```python
from build123d import *

# Parameters (mm, degrees)
SKETCH1_W               = 700
SKETCH1_H               = 450
BOSS_EXTRUDE1_DEPTH     = 1000
SKETCH2_W               = 650
SKETCH2_H               = 600
CUT_EXTRUDE1_DEPTH      = 250
CUT_EXTRUDE1_DEPTH_BACK = 250
SKETCH3_W               = 650
SKETCH3_H               = 350
CUT_EXTRUDE2_DEPTH      = 250
CUT_EXTRUDE2_DEPTH_BACK = 250
SKETCH4_W               = 400
SKETCH4_H               = 600
CUT_EXTRUDE3_DEPTH      = 400
CUT_EXTRUDE3_DEPTH_BACK = 400
SKETCH5_W               = 400
SKETCH5_H               = 350
CUT_EXTRUDE4_DEPTH      = 400
CUT_EXTRUDE4_DEPTH_BACK = 400
ESBO_O1_R               = 8
ESBO_O1_W               = 150
ESBO_O1_H               = 110
CORTE_EXTRUS_O1_DEPTH   = 50
ESBO_O2_W               = 250
ESBO_O2_H               = 70
CORTE_EXTRUS_O2_DEPTH   = 26
ESBO_O3_R               = 6.25
CORTE_EXTRUS_O3_DEPTH   = 10
ESBO_O5_R               = 3
CORTE_EXTRUS_O4_DEPTH   = 26
ESBO_O7_R               = 6
CORTE_EXTRUS_O5_DEPTH   = 5


with BuildPart() as part:
    # Sketch1 → Boss-Extrude1 (new body)
    with BuildSketch(Plane(origin=(0, 0, 0), x_dir=(1, 0, 0), z_dir=(0, 1, 0))):
        Rectangle(SKETCH1_W, SKETCH1_H)
    extrude(amount=BOSS_EXTRUDE1_DEPTH)

    # Sketch2 → Cut-Extrude1 (cut, two sides)
    with BuildSketch(Plane.XY) as cut_extrude1_sk:
        with Locations((0, 675)):
            Rectangle(SKETCH2_W, SKETCH2_H)
    extrude(amount=CUT_EXTRUDE1_DEPTH, mode=Mode.SUBTRACT)
    extrude(cut_extrude1_sk.sketch, amount=-CUT_EXTRUDE1_DEPTH_BACK, mode=Mode.SUBTRACT)

    # Sketch3 → Cut-Extrude2 (cut, two sides)
    with BuildSketch(Plane.XY) as cut_extrude2_sk:
        with Locations((0, 175)):
            Rectangle(SKETCH3_W, SKETCH3_H)
    extrude(amount=CUT_EXTRUDE2_DEPTH, mode=Mode.SUBTRACT)
    extrude(cut_extrude2_sk.sketch, amount=-CUT_EXTRUDE2_DEPTH_BACK, mode=Mode.SUBTRACT)

    # Sketch4 → Cut-Extrude3 (cut, two sides)
    with BuildSketch(Plane(origin=(0, 0, 0), x_dir=(0, 0, -1), z_dir=(1, 0, 0))) as cut_extrude3_sk:
        with Locations((0, 675)):
            Rectangle(SKETCH4_W, SKETCH4_H)
    extrude(amount=CUT_EXTRUDE3_DEPTH, mode=Mode.SUBTRACT)
    extrude(cut_extrude3_sk.sketch, amount=-CUT_EXTRUDE3_DEPTH_BACK, mode=Mode.SUBTRACT)

    # Sketch5 → Cut-Extrude4 (cut, two sides)
    with BuildSketch(Plane(origin=(0, 0, 0), x_dir=(0, 0, -1), z_dir=(1, 0, 0))) as cut_extrude4_sk:
        with Locations((0, 175)):
            Rectangle(SKETCH5_W, SKETCH5_H)
    extrude(amount=CUT_EXTRUDE4_DEPTH, mode=Mode.SUBTRACT)
    extrude(cut_extrude4_sk.sketch, amount=-CUT_EXTRUDE4_DEPTH_BACK, mode=Mode.SUBTRACT)

    # Esboço1 → Corte-extrusão1 (cut)
    with BuildSketch(Plane(origin=(0, 1000, 0), x_dir=(1, 0, 0), z_dir=(0, 1, 0))):
        with Locations((-100.84, 100)):
            Circle(ESBO_O1_R)
        with Locations((-230, 100)):
            Circle(ESBO_O1_R)
        with Locations((-230, -74.37)):
            Circle(ESBO_O1_R)
        with Locations((0, -74.37)):
            Circle(ESBO_O1_R)
        with Locations((230, -74.37)):
            Circle(ESBO_O1_R)
        with Locations((-165.42, 10.42)):
            Rectangle(ESBO_O1_W, ESBO_O1_H)
    extrude(amount=-CORTE_EXTRUS_O1_DEPTH, mode=Mode.SUBTRACT)

    # Esboço2 → Corte-extrusão2 (cut, through all)
    with BuildSketch(Plane(origin=(0, 975, 0), x_dir=(-1, 0, 0), z_dir=(0, -1, 0))):
        with Locations((-170, -105)):
            Rectangle(ESBO_O2_W, ESBO_O2_H)
    extrude(amount=-CORTE_EXTRUS_O2_DEPTH, mode=Mode.SUBTRACT)

    # Esboço3 → Corte-extrusão3 (cut)
    with BuildSketch(Plane(origin=(0, 1000, 0), x_dir=(1, 0, 0), z_dir=(0, 1, 0))):
        with Locations((270, -13.671274916)):
            Circle(ESBO_O3_R)
        with Locations((270, 96.328725084)):
            Circle(ESBO_O3_R)
        with Locations((125, 96.328725084)):
            Circle(ESBO_O3_R)
        with Locations((125, -13.671274916)):
            Circle(ESBO_O3_R)
    extrude(amount=-CORTE_EXTRUS_O3_DEPTH, mode=Mode.SUBTRACT)

    # Esboço5 → Corte-extrusão4 (cut, through all)
    with BuildSketch(Plane.XZ.offset(-975)):
        with Locations((93, -180)):
            Circle(ESBO_O5_R)
        with Locations((93, -113.3)):
            Circle(ESBO_O5_R)
        with Locations((230, -113.3)):
            Circle(ESBO_O5_R)
        with Locations((230, -180)):
            Circle(ESBO_O5_R)
    extrude(amount=-CORTE_EXTRUS_O4_DEPTH, mode=Mode.SUBTRACT)

    # Esboço7 → Corte-extrusão5 (cut)
    with BuildSketch(Plane(origin=(0, 1000, 0), x_dir=(1, 0, 0), z_dir=(0, 1, 0))):
        with Locations((315, 75)):
            Circle(ESBO_O7_R)
    extrude(amount=-CORTE_EXTRUS_O5_DEPTH, mode=Mode.SUBTRACT)


solid = part.part
```
Design review of the part built by this model. Coordinates are the model's own, in mm. A direction names the side the tool comes from. Coordinates: 2 decimals unless noted, no trailing zeros. Write each loop counter-clockwise with the first axis right and the second up, starting at its lowest first coordinate (ties: lowest second). Pieces come first, ordered by that corner, then holes.
1) To check wall thickness, follow L1, parallel to Z at x = 230, y = 987.25; L2, parallel to Z at x = 315, y = 998; L3, parallel to X at y = 991.25, z = 74.37. State the ranges of each line that lie inside material, in increasing order.
2) Add section A-A (x = -169.5). Write out the cut boundary in (y, z).
3) Insertion check: pin 1 (21 mm diameter, centred on x = -100.84, z = -100, fed in from -Y); pin 2 (4 mm diameter, centred on x = 267.5, z = 15.5, fed in from +Y). Each pin has a flat end and moves straight along its axis. Give the tip position at first contact, or say it passes through.
4) Add section D-D (y = 730). Write out the cut boundary in (x, z), plus the area to 3 significant figures.
5) Machinability: for faces 1 (the flat face through (-337, 173, -200)), 2 (the flat face through (337, 671, -200)), 3 (the flat face through (325, 671, 212)), which of the approach directions +Z, -Z, +X, -X, +Y, -Y give a long, thin tool a straight path to every point of the face, cutting with its end or side? Answer none if there is none.
6) Add section B-B (x = -74.5). Write out the cut boundary in (y, z), plus the area to 3 significant figures.
7) Add section C-C (z = 102.5). Write out the cut boundary in (x, y).
8) Mouldability with a two-part tool opening along Y and no side actions: class faces 4 (the flat face through (-337, 671, -200)), 5 (the flat face through (-338, 0, 212)), 6 (the flat face through (337, 173, -200)) as +Y half, -Y half, draft (parallel to the pull), parting line (faces both ways), or undercut.
Check result:
1. L1: z = -225 to -183, -177 to -116.3, -110.3 to 66.37, 140 to 225
1. L2: z = -225 to -81, -69 to 225
1. L3: x = -350 to -238, -222 to -8, 8 to 45, 295 to 350
2. outline: (350, -225) - (375, -225) - (375, 225) - (350, 225) - close; (975, -225) - (1000, -225) - (1000, -65.42) - (975, -65.42) - close; (975, 44.58) - (1000, 44.58) - (1000, 225) - (975, 225) - close
3. pin 1: stops at y = 350
3. pin 2: stops at y = 990
4. outline: (-350, -225) - (-325, -225) - (-325, -200) - (-350, -200) - close; (-350, 200) - (-325, 200) - (-325, 225) - (-350, 225) - close; (325, -225) - (350, -225) - (350, -200) - (325, -200) - close; (325, 200) - (350, 200) - (350, 225) - (325, 225) - close
4. area: 2,500 mm2
5. face 1: +X, -X, -Y
5. face 2: +X, -X
5. face 3: +Z, -Z
6. outline: (350, -225) - (375, -225) - (375, 225) - (350, 225) - close; (975, -225) - (1000, -225) - (1000, 225) - (975, 225) - close
6. area: 22,500 mm2
7. outline: (-350, 350) - (350, 350) - (350, 375) - (-350, 375) - close; (-350, 975) - (45, 975) - (45, 1000) - (-350, 1000) - close; (295, 975) - (350, 975) - (350, 1000) - (295, 1000) - close
8. face 4: undercut
8. face 5: -Y half
8. face 6: draft
